from build123d import *

# Parameters (mm, degrees)
BOSS_EXTRUDE1_DEPTH = 1
SKETCH3_R           = 4.5
SKETCH3_R_2         = 3.5
BOSS_EXTRUDE2_DEPTH = 2.2
SKETCH4_R           = 1.4
BOSS_EXTRUDE3_DEPTH = 3


with BuildPart() as part:
    # Sketch1 → Boss-Extrude1 (new body)
    with BuildSketch(Plane.XY):
        with BuildLine():
            Line((-9.526279442, -5.5), (9.526279442, -5.5))
            ThreePointArc((9.526279442, -5.5), (0, 11), (-9.526279442, -5.5))
        make_face()
    extrude(amount=BOSS_EXTRUDE1_DEPTH)

    # Sketch3 → Boss-Extrude2 (add)
    with BuildSketch(Plane(origin=(0, 0, 0), x_dir=(-1, 0, 0), z_dir=(0, 0, -1))):
        Circle(SKETCH3_R)
        Circle(SKETCH3_R_2, mode=Mode.SUBTRACT)
    extrude(amount=BOSS_EXTRUDE2_DEPTH)

    # Sketch4 → Boss-Extrude3 (add)
    with BuildSketch(Plane(origin=(0, 0, 0), x_dir=(-1, 0, 0), z_dir=(0, 0, -1))):
        Circle(SKETCH4_R)
    extrude(amount=BOSS_EXTRUDE3_DEPTH)


solid = part.part
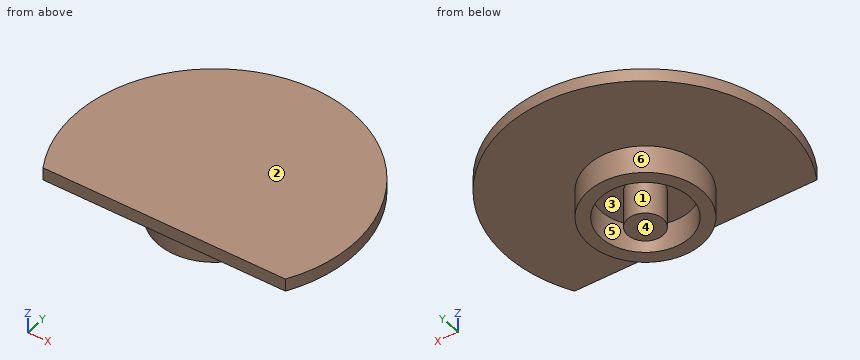
For this review, take the finished solid that the model builds, in its own axes (mm). Face numbers are marked on the shaded views. A direction names the side the tool comes from. Round coordinates to 2 decimals unless told otherwise and drop trailing zeros. Order: outer loops, then holes, each group sorted by start corner. A loop starts at its lowest first (then second) coordinate and runs counter-clockwise, first axis right, second up. Notation, with made-up numbers: M -8,72 L 14,72 A30 ccw 14,94 Z; hole C -32,8.5 d6. An arc over 180 degrees is marked long. Use a Markdown table: item, result. Add a question column.
Item 1: Add section B-B, the plane y = 0. Give the boundary of the cut face in (x, z), then the cut area to 3 significant figures.
Item 2: Add section D-D, the plane x = -2.25. Give the boundary of the cut face in (y, z).
Item 3: Add section C-C, the plane x = 0. Give the boundary of the cut face in (y, z).
Item 4: Insertion check: pin 1 (1 mm diameter, centred on x = -2, z = -1.5, fed in from -Y); pin 2 (2.5 mm diameter, centred on x = 0.5, y = -1.5, fed in from -Z); pin 3 (1.5 mm diameter, centred on y = 3, z = -1.5, fed in from -X). Each pin has a flat end and moves straight along its axis. Give the tip position at first contact, or say it passes through.
Item 5: To check wall thickness, follow line 1 along Y through (x, z) = (0, -1.1); line 2 along Y through (x, z) = (1.25, -1.75); line 3 along Z through (x, y) = (-5.25, -4.5). State the ranges of each line that lie inside material, in increasing order.
Item 6: Add section A-A, the plane z = -1.3. Give the boundary of the cut face in (x, y).
Item 7: Mouldability with a two-part tool opening along Y and no side actions: class the marked faces 3, 4, 5 and 6 as released by +Y, released by -Y, zero draft, split by the parting line, or undercut.
Item 8: Tool access review of the marked faces 1 and 2: name each direction out of +Z, -Z, +X, -X, +Y, -Y from which nothing blocks a thin tool from reaching the whole face with its end or side.
Geometry results:
| question | item | result |
|---|---|---|
| 1 | outline | M -11,0 L -4.5,0 L -4.5,-2.2 L -3.5,-2.2 L -3.5,0 L -1.4,0 L -1.4,-3 L 1.4,-3 L 1.4,0 L 3.5,0 L 3.5,-2.2 L 4.5,-2.2 L 4.5,0 L 11,0 L 11,1 L -11,1 Z |
| 1 | area | 34.8 mm² |
| 2 | outline | M -5.5,0 L -3.9,0 L -3.9,-2.2 L -2.68,-2.2 L -2.68,0 L 2.68,0 L 2.68,-2.2 L 3.9,-2.2 L 3.9,0 L 10.77,0 L 10.77,1 L -5.5,1 Z |
| 3 | outline | M -5.5,0 L -4.5,0 L -4.5,-2.2 L -3.5,-2.2 L -3.5,0 L -1.4,0 L -1.4,-3 L 1.4,-3 L 1.4,0 L 3.5,0 L 3.5,-2.2 L 4.5,-2.2 L 4.5,0 L 11,0 L 11,1 L -5.5,1 Z |
| 4 | pin 1 | stops at y = -4.24 |
| 4 | pin 2 | stops at z = -3 |
| 4 | pin 3 | stops at x = -3.9 |
| 5 | line 1 | y = -4.5 to -3.5, -1.4 to 1.4, 3.5 to 4.5 |
| 5 | line 2 | y = -4.32 to -3.27, -0.63 to 0.63, 3.27 to 4.32 |
| 5 | line 3 | z = 0 to 1 |
| 6 | outline | C 0,0 d9; C 0,0 d2.8; hole C 0,0 d7 |
| 7 | face 3 | undercut |
| 7 | face 4 | zero draft |
| 7 | face 5 | undercut |
| 7 | face 6 | split by the parting line |
| 8 | face 1 | -Z |
| 8 | face 2 | +Z, +X, -X, +Y, -Y |
